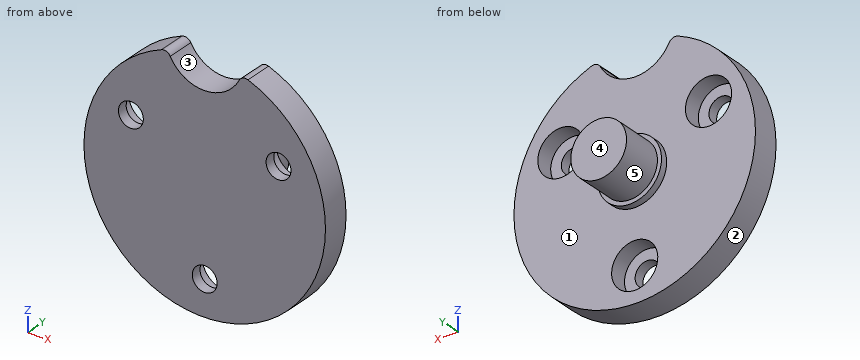
```python
from build123d import *

# Parameters (mm, degrees)
SKETCH1_R           = 17
SKETCH1_R_2         = 1.75
BOSS_EXTRUDE1_DEPTH = 4
SKETCH2_R           = 3.25
CUT_EXTRUDE1_DEPTH  = 2.5
SKETCH3_R           = 4.5
BOSS_EXTRUDE2_DEPTH = 1
SKETCH4_R           = 3.925
BOSS_EXTRUDE3_DEPTH = 6
CUT_EXTRUDE2_REACH  = 27.04
SKETCH5_R           = 5.5
FILLET1_R           = 1


with BuildPart() as part:
    # Sketch1 → Boss-Extrude1 (new body)
    with BuildSketch(Plane(origin=(0, 0, 0), x_dir=(1, 0, 0), z_dir=(0, 1, 0))):
        with Locations(Location((0, 0, 0), (0, 0, 270))):
            Circle(SKETCH1_R)
        with Locations(Location((0, 12, 0), (0, 0, 270))):
            Circle(SKETCH1_R_2, mode=Mode.SUBTRACT)
        with Locations(Location((10.392304845, -6, 0), (0, 0, 270))):
            Circle(SKETCH1_R_2, mode=Mode.SUBTRACT)
        with Locations(Location((-10.392304845, -6, 0), (0, 0, 270))):
            Circle(SKETCH1_R_2, mode=Mode.SUBTRACT)
    extrude(amount=BOSS_EXTRUDE1_DEPTH)

    # Sketch2 → Cut-Extrude1 (cut)
    with BuildSketch(Plane(origin=(0, 4, 0), x_dir=(1, 0, 0), z_dir=(0, 1, 0))):
        with Locations(Location((0, 12, 0), (0, 0, 270))):
            Circle(SKETCH2_R)
        with Locations(Location((10.392304845, -6, 0), (0, 0, 270))):
            Circle(SKETCH2_R)
        with Locations(Location((-10.392304845, -6, 0), (0, 0, 270))):
            Circle(SKETCH2_R)
    extrude(amount=-CUT_EXTRUDE1_DEPTH, mode=Mode.SUBTRACT)

    # Sketch3 → Boss-Extrude2 (add)
    with BuildSketch(Plane(origin=(0, 4, 0), x_dir=(1, 0, 0), z_dir=(0, 1, 0))):
        with Locations(Location((0, 0, 0), (0, 0, 270))):
            Circle(SKETCH3_R)
    extrude(amount=BOSS_EXTRUDE2_DEPTH)

    # Sketch4 → Boss-Extrude3 (add)
    with BuildSketch(Plane(origin=(0, 5, 0), x_dir=(1, 0, 0), z_dir=(0, 1, 0))):
        with Locations(Location((0, 0, 0), (0, 0, 270))):
            Circle(SKETCH4_R)
    extrude(amount=BOSS_EXTRUDE3_DEPTH)

    # Sketch5 → Cut-Extrude2 (cut, up to next)
    with BuildSketch(Plane(origin=(0, 4, 0), x_dir=(1, 0, 0), z_dir=(0, 1, 0)), mode=Mode.PRIVATE) as cut_extrude2_sk1:
        with Locations((0, -18)):
            Circle(SKETCH5_R)
    cut_extrude2_tool1 = extrude(cut_extrude2_sk1.sketch, amount=-CUT_EXTRUDE2_REACH, mode=Mode.PRIVATE) & part.part
    add(cut_extrude2_tool1.solids().sort_by_distance((0, 4, 18))[0], mode=Mode.SUBTRACT)

    # Fillet1
    fillet1_edges = [part.edges().sort_by_distance(p)[0] for p in [
        (-5.192768409, 2, 16.1875),
        (5.192768409, 2, 16.1875),
    ]]
    fillet(fillet1_edges, radius=FILLET1_R)


solid = part.part
```
Check sheet for the modelled part. Datum: model origin and axes. Units: mm. Face numbers are marked on the shaded views. A direction names the side the tool comes from. Coordinates: 2 decimals unless noted, no trailing zeros. Order: outer loops, then holes, each group sorted by start corner. A loop starts at its lowest first (then second) coordinate and runs counter-clockwise, first axis right, second up. Notation, with made-up numbers: (-8, 28) -> (20, 28) arc R19 ccw to (20, 59) -> close; hole circle Ø9 at (26, 75). An arc over 180 degrees is marked (long way). Write item = value, one per line. Start each with the question number.
1) Mould release check, pull along X, two halves, no side actions. Record for the marked faces 1, 2 and 3: +X half, -X half, draft (parallel to the pull), parting line (faces both ways), or undercut.
2) Cross-section at C-C (z = 6). Enter the section's corners in (x, y), then the cut area to 3 significant figures.
3) Material ranges on L1, parallel to X at y = 0.35, z = 6; L2, parallel to Y at x = -5.5, z = -12.5; L3, parallel to Y at x = 12.5, z = 6.5, recorded low to high.
4) Access from +Z, -Z, +X, -X, +Y, -Y to the whole of each face (thin tool, end or side, straight path). Record for the marked faces 4 and 5.
5) Go/stop test with flat-tipped pins: P1, Ø2, axis at x = -10.5, z = 7.5, coming from the +Y side; P2, Ø4, axis at x = 0, z = -12, coming from the -Y side; P3, Ø5, axis at x = -1, z = -13.5, coming from the +Y side; P4, Ø1.5, axis at x = -11, y = 2, coming from the +Z side. Record where each tip stops, or that it passes through.
6) Cross-section at B-B (z = -12). Enter the section's corners in (x, y), then the cut area to 3 significant figures.
7) Cross-section at D-D (z = 0). Enter the section's corners in (x, y) (3 decimals).
8) Cross-section at A-A (x = 0). Enter the section's corners in (y, z) (3 decimals), then the cut area to 3 significant figures.
Ans:
q1.face_1 = draft
q1.face_2 = parting line
q1.face_3 = undercut
q2.outline = (-15.91, 0) -> (-12.14, 0) -> (-12.14, 1.5) -> (-13.64, 1.5) -> (-13.64, 4) -> (-15.91, 4) -> close; (-8.64, 0) -> (8.64, 0) -> (8.64, 1.5) -> (7.14, 1.5) -> (7.14, 4) -> (-7.14, 4) -> (-7.14, 1.5) -> (-8.64, 1.5) -> close; (12.14, 0) -> (15.91, 0) -> (15.91, 4) -> (13.64, 4) -> (13.64, 1.5) -> (12.14, 1.5) -> close
q2.area = 84.2 mm²
q3.L1 = -15.91 to -12.14, -8.64 to 8.64, 12.14 to 15.91
q3.L2 = 0 to 4
q3.L3 = 0 to 1.5
q4.face_4 = +Z, -Z, +X, -X, +Y
q4.face_5 = +Y
q5.P1 = 1.5
q5.P2 = 0
q5.P3 = 4
q5.P4 = 13.56
q6.outline = (-12.04, 0) -> (-1.75, 0) -> (-1.75, 1.5) -> (-3.25, 1.5) -> (-3.25, 4) -> (-12.04, 4) -> close; (1.75, 0) -> (12.04, 0) -> (12.04, 4) -> (3.25, 4) -> (3.25, 1.5) -> (1.75, 1.5) -> close
q6.area = 74.8 mm²
q7.outline = (-17, 0) -> (17, 0) -> (17, 4) -> (4.5, 4) -> (4.5, 5) -> (3.925, 5) -> (3.925, 11) -> (-3.925, 11) -> (-3.925, 5) -> (-4.5, 5) -> (-4.5, 4) -> (-17, 4) -> close
q8.outline = (0, -17) -> (4, -17) -> (4, -15.25) -> (1.5, -15.25) -> (1.5, -13.75) -> (0, -13.75) -> close; (0, -10.25) -> (1.5, -10.25) -> (1.5, -8.75) -> (4, -8.75) -> (4, -4.5) -> (5, -4.5) -> (5, -3.925) -> (11, -3.925) -> (11, 3.925) -> (5, 3.925) -> (5, 4.5) -> (4, 4.5) -> (4, 12.5) -> (0, 12.5) -> close
q8.area = 153 mm²
